```python
from build123d import *

# Parameters (mm, degrees)
SKETCH_1_R             = 5
EXTRUDE_1_DEPTH        = 1.9
SKETCH_2_R             = 2.5
EXTRUDE_2_DEPTH        = 27
HOLE_WIZARD_M4_1_D     = 3.3
HOLE_WIZARD_M4_1_DEPTH = 10.1
HOLE_WIZARD_M4_1_TIP   = 0.991420021
CHAMFER_1_SIZE         = 0.5
CHAMFER_1_SIZE2        = 0.866025404


with BuildPart() as part:
    # 草图1 → 凸台-拉伸1 (new body)
    with BuildSketch(Plane(origin=(0, 0, 0), x_dir=(0, 0, -1), z_dir=(1, 0, 0))):
        with Locations(Location((0, 0, 0), (0, 0, 180))):
            Circle(SKETCH_1_R)
    extrude(amount=EXTRUDE_1_DEPTH)

    # 草图2 → 凸台-拉伸2 (add)
    with BuildSketch(Plane(origin=(1.9, 0, 0), x_dir=(0, 0, -1), z_dir=(1, 0, 0))):
        Circle(SKETCH_2_R)
    extrude(amount=EXTRUDE_2_DEPTH)

    # M4 螺纹孔1
    with Locations(Plane(origin=(28.9, 0, 0), x_dir=(0, 0, 1), z_dir=(1, 0, 0))):
        with Locations((0, 0)):
            Hole(HOLE_WIZARD_M4_1_D / 2, depth=HOLE_WIZARD_M4_1_DEPTH)
            with Locations((0, 0, -(HOLE_WIZARD_M4_1_DEPTH + HOLE_WIZARD_M4_1_TIP / 2))):  # 118° drill point
                Cone(0, HOLE_WIZARD_M4_1_D / 2, HOLE_WIZARD_M4_1_TIP, mode=Mode.SUBTRACT)

    # 倒角1
    chamfer_1_edges = [part.edges().sort_by_distance(p)[0] for p in [
        (0, 0, -5),
    ]]
    chamfer_1_side = [part.faces().sort_by_distance(p)[0] for p in [
        (0.95, 0, -5),
    ]]
    chamfer(chamfer_1_edges, length=CHAMFER_1_SIZE, length2=CHAMFER_1_SIZE2, reference=chamfer_1_side[0])


solid = part.part
```
Read the model definition and answer for the solid it produces. Units are mm, in the model's axes. A direction names the side the tool comes from. Round coordinates to 2 decimals unless told otherwise and drop trailing zeros. Write each loop counter-clockwise with the first axis right and the second up, starting at its lowest first coordinate (ties: lowest second). Pieces come first, ordered by that corner, then holes. Notation, with made-up numbers: (48.25, 49) - (84.25, 49) arc R21 ccw to (84.25, 59) - close; hole circle Ø10 at (-32, 80). An arc over 180 degrees is marked (long way). Use CSV: the item, a comma, the result in double quotes.
Q1. Find section B-B, the plane x = 15. Write down the section's boundary in (y, z), then the cut area to 3 significant figures.
Values:
outline,"circle Ø5 at (0, 0)"
area,"19.6 mm²"
Q2. Straight lines are drawn through the part: line 1 along Y through (x, z) = (26.5, 0); line 2 along X through (y, z) = (3.5, 1.25); line 3 along Y through (x, z) = (21, 1). For each, find the intervals that lie inside material, in ascending order.
Values:
line 1,"y = -2.5 to -1.65, 1.65 to 2.5"
line 2,"x = 0 to 1.9"
line 3,"y = -2.29 to -1.31, 1.31 to 2.29"
Q3. Each of these flat-tipped pins is pushed along its axis until it touches: pin 1 Ø3 at (y, z) = (0, 0) entering from +X; pin 2 Ø2 at (x, y) = (23, -1) entering from -Z; pin 3 Ø1.5 at (x, y) = (14.5, 1) entering from +Z. Where does it stop, or does it pass through?
Values:
pin 1,"stops at x = 18.71"
pin 2,"stops at z = -2.5"
pin 3,"stops at z = 2.49"
Q4. Find section A-A, the plane x = 24. Write down the section's boundary in (y, z).
Values:
outline,"circle Ø5 at (0, 0); hole circle Ø3.3 at (0, 0)"
Q5. A tool of negligible diameter and unlimited length cuts with its end or side. For faces 4 (the cylindrical face through (23.779, -1.115, 1.216)), 5 (the cylindrical face through (1, 0, -5)), from which of +Z, -Z, +X, -X, +Y, -Y can it reach the whole face along a straight path? Write none if from no direction.
Values:
face 4,"+X"
face 5,"+X, -X"
Q6. Determine the mould class of faces 1 (the conical face through (18, 0.1, 0.3)), 2 (the flat face through (0, 0, 0)), 3 (the cylindrical face through (15.21, -2.44, 0.54)) for opening direction Y: +Y half, -Y half, draft (parallel to the pull), parting line (faces both ways), or undercut.
Values:
face 1,"undercut"
face 2,"draft"
face 3,"parting line"
